Autodesk Inventor part; units mm, degrees
ref_plane "YZ Plane" through (0, 0, 0) normal (1, 0, 0) x (0, 1, 0)
ref_plane "XZ Plane" through (0, 0, 0) normal (0, 1, 0) x (-1, 0, 0)
ref_plane "XY Plane" through (0, 0, 0) normal (0, 0, 1) x (1, 0, 0)
sketch "Sketch1" plane through (0, 0, 0) normal (0, 0, 1) x (1, 0, 0)
  circle A0 centre (-21.9525, -0.0633) radius 1
  circle A1 centre (22.0475, -0.0633) radius 1
  circle A2 centre (-21.9525, -0.0633) radius 1.125
  circle A3 centre (22.0475, -0.0633) radius 1.125
  circle A4 centre (-21.9525, -0.0633) radius 3
  circle A5 centre (22.0475, -0.0633) radius 3
  line L0 (-21.9525, 2.9367) -> (22.0475, 2.9367)
  line L1 (-21.9525, -3.0633) -> (22.0475, -3.0633)
  point P0 (0, 0)
  dimension "d0" = 2.25
  dimension "d1" = 2.25
  dimension "d2" = 6
  dimension "d3" = 6
extrude "Extrusion1" add sketch "Sketch1" along normal blind 4 contours A4 | A4 L0 A5 L1 | A5
properties part number "servostrap_3DPrint"
Model file for the job. Use its own axes, mm. Give positions to 0.01 mm unless a question says otherwise; leave off trailing zeros. Loops run counter-clockwise (first coordinate to the right, second up) from the corner with the lowest first, then second, coordinate; pieces in that order, holes last.
1) Saw through at D-D (y = -2.5). Write the cut outline in (x, z).
2) Wall check: line 1 (X direction, y = 0, z = 3.75); line 2 (X direction, y = -0.3, z = 3.5); line 3 (X direction, y = -1.55, z = 2.75). Give the ranges that are in metal, low to high.
3) Saw through at B-B (z = 1.45). Count the separate pieces of the cut face and the enclosed holes in it, plus the area to 3 significant figures.
4) Pull direction X, two halves, no side cores. Call faces 1 (the flat face through (0, -3.063, 2)), 2 (the cylindrical face through (-24.95, -0.13, 1.97)), 3 (the cylindrical face through (-23.076, -0.113, 1.972)): +X half, -X half, draft (parallel to the pull), parting line (faces both ways), or undercut.
5) Saw through at C-C (y = 1.7). Write the cut outline in (x, z), plus the area to 3 significant figures.
6) Saw through at A-A (y = -0.7). Write the cut outline in (x, z) (3 decimals).
Answer block:
1. outline: (-23.7, 0) - (23.8, 0) - (23.8, 4) - (-23.7, 4) - close
2. line 1: x = -24.95 to -23.08, -20.83 to 20.92, 23.17 to 25.05
2. line 2: x = -24.94 to -23.05, -20.85 to 20.95, 23.15 to 25.04
2. line 3: x = -24.56 to 24.65
3. separate pieces: 1
3. enclosed holes: 2
3. area: 284 mm2
4. face 1: draft
4. face 2: -X half
4. face 3: undercut
5. outline: (-24.38, 0) - (24.47, 0) - (24.47, 4) - (-24.38, 4) - close
5. area: 195 mm2
6. outline: (-24.884, 0) - (-22.88, 0) - (-22.88, 4) - (-24.884, 4) - close; (-21.025, 0) - (21.12, 0) - (21.12, 4) - (-21.025, 4) - close; (22.975, 0) - (24.979, 0) - (24.979, 4) - (22.975, 4) - close
